Can you work these out from the drawing? Everything is in mm from the part's minimum corner. A direction names the side the tool comes from. Give positions to 0.01 mm unless a question says otherwise; leave off trailing zeros. Loops run counter-clockwise (first coordinate to the right, second up) from the corner with the lowest first, then second, coordinate; pieces in that order, holes last. Notation, with made-up numbers: (40, 14) - (94, 14) arc R32 cw to (94, 49) - close; hole circle Ø7 at (55.5, 25.25). An arc over 180 degrees is marked (long way). Answer in a Markdown table with one row per item.
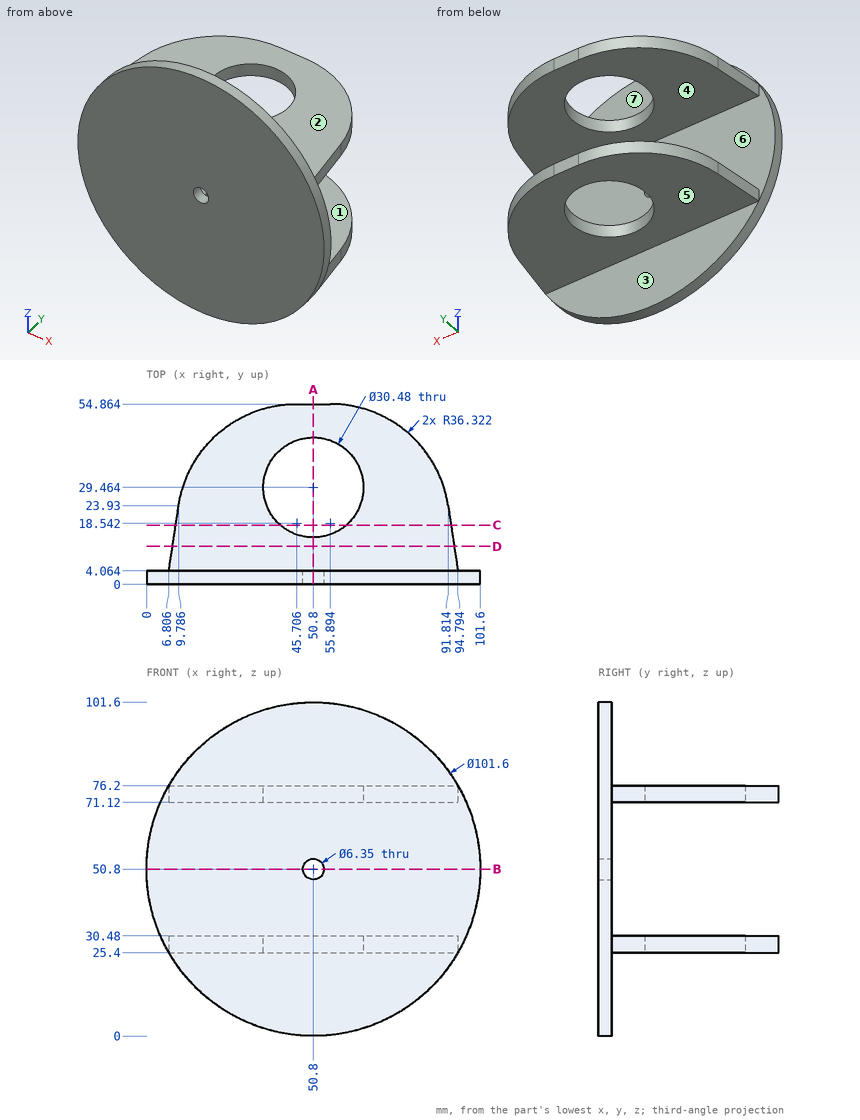
Q1. Imagine slicing it at D-D, the plane y = 11.5. Write out the boundary of the cut face in (x, z), and give its area (3 significant figures).
Checked values:
| item | result |
|---|---|
| outline | (7.92, 25.4) - (93.68, 25.4) - (93.68, 30.48) - (7.92, 30.48) - close; (7.92, 71.12) - (93.68, 71.12) - (93.68, 76.2) - (7.92, 76.2) - close |
| area | 871 mm² |
Q2. For pin 1 (8 mm diameter, centred on x = 39.5, y = 25.5, fed in from +Z); pin 2 (8.5 mm diameter, centred on x = 50.8, z = 50.8, fed in from +Y); pin 3 (8 mm diameter, centred on y = 11, z = 36, fed in from +X); pin 4 (2 mm diameter, centred on y = 6, z = 75, fed in from +X), each with a flat end and sliding along its axis, tell me the tip position at first contact or that it passes through.
Checked values:
| item | result |
|---|---|
| pin 1 | stops at z = 76.2 |
| pin 2 | stops at y = 4.06 |
| pin 3 | passes through |
| pin 4 | stops at x = 94.65 |
Q3. On a 3-axis mill with a long thin cutter (end or side, diameter ignored), from which of +Z, -Z, +X, -X, +Y, -Y can I reach the whole of each face in a straight line? I mean the marked faces 1, 2 and 3. Say none if no direction works.
Checked values:
| item | result |
|---|---|
| face 1 | +X, -X, +Y |
| face 2 | +Z, +X, -X, +Y |
| face 3 | -Z, +X, -X, +Y |
Q4. Imagine slicing it at B-B, the plane z = 50.8. Write out the boundary of the cut face in (x, y) (3 decimals).
Checked values:
| item | result |
|---|---|
| outline | (0, 0) - (47.625, 0) - (47.625, 4.064) - (0, 4.064) - close; (53.975, 0) - (101.6, 0) - (101.6, 4.064) - (53.975, 4.064) - close |
Q5. Imagine slicing it at C-C, the plane y = 18. Write out the boundary of the cut face in (x, z).
Checked values:
| item | result |
|---|---|
| outline | (8.9, 25.4) - (40.76, 25.4) - (40.76, 30.48) - (8.9, 30.48) - close; (8.9, 71.12) - (40.76, 71.12) - (40.76, 76.2) - (8.9, 76.2) - close; (60.84, 25.4) - (92.7, 25.4) - (92.7, 30.48) - (60.84, 30.48) - close; (60.84, 71.12) - (92.7, 71.12) - (92.7, 76.2) - (60.84, 76.2) - close |
Q6. If I drill on line 1 (Y direction, x = 50.8, z = 74.5); line 2 (Z direction, x = 18.5, y = 7.5); line 3 (Z direction, x = 50.8, y = 2.6) (3 decimals), over which ranges is the centre line in solid material (lowest first)? Write a range as [from, to].
Checked values:
| item | result |
|---|---|
| line 1 | y = [0, 14.22], [44.7, 54.86] |
| line 2 | z = [25.4, 30.48], [71.12, 76.2] |
| line 3 | z = [0, 47.625], [53.975, 101.6] |
Q7. Imagine slicing it at A-A, the plane x = 50.8. Write out the boundary of the cut face in (y, z) (3 decimals).
Checked values:
| item | result |
|---|---|
| outline | (0, 0) - (4.064, 0) - (4.064, 25.4) - (14.224, 25.4) - (14.224, 30.48) - (4.064, 30.48) - (4.064, 47.625) - (0, 47.625) - close; (0, 53.975) - (4.064, 53.975) - (4.064, 71.12) - (14.224, 71.12) - (14.224, 76.2) - (4.064, 76.2) - (4.064, 101.6) - (0, 101.6) - close; (44.704, 25.4) - (54.864, 25.4) - (54.864, 30.48) - (44.704, 30.48) - close; (44.704, 71.12) - (54.864, 71.12) - (54.864, 76.2) - (44.704, 76.2) - close |
Q8. If we mould it in two halves opening along Z, with no side actions, what happens to the marked faces 4, 5, 6 and 7? For each: released by +Z, released by -Z, zero draft, split by the parting line, or undercut.
Checked values:
| item | result |
|---|---|
| face 4 | undercut |
| face 5 | released by -Z |
| face 6 | undercut |
| face 7 | zero draft |
